from build123d import *

# Parameters (mm, degrees)
SKETCH3_W           = 6
SKETCH3_H           = 5
BOSS_EXTRUDE6_DEPTH = 6
CUT_EXTRUDE3_DEPTH  = 3


with BuildPart() as part:
    # Sketch3 → Boss-Extrude6 (new body)
    with BuildSketch(Plane.XY):
        with Locations((3, 2.5)):
            Rectangle(SKETCH3_W, SKETCH3_H)
    extrude(amount=BOSS_EXTRUDE6_DEPTH)

    # Sketch7 → Cut-Extrude3 (cut)
    with BuildSketch(Plane.ZY):
        Polygon((0, 5), (6, 3), (6, 5), align=None)
    extrude(amount=-CUT_EXTRUDE3_DEPTH, mode=Mode.SUBTRACT)


solid = part.part
Input: part model. Units: mm. Frame: model coordinates. A direction names the side the tool comes from. Round coordinates to 2 decimals unless told otherwise and drop trailing zeros. Loops run counter-clockwise (first coordinate to the right, second up) from the corner with the lowest first, then second, coordinate; pieces in that order, holes last. Notation, with made-up numbers: (-18.5, -12) -> (11.5, -12) arc R22 cw to (11.5, 18) -> close; hole circle Ø9 at (71, -39). An arc over 180 degrees is marked (long way). Answer as a JSON object with one key per item and string values. Group by question number.
1) Reachability of faces 1 (the flat face through (4, 2, 6)), 2 (the flat face through (3, 4, 4)) from +Z, -Z, +X, -X, +Y, -Y: full face, straight path, thin tool, end or side. Return the list, or none.
2) Section query B-B on z = 0.75. Output: boundary loops of the cut face in (x, y).
3) Section query C-C on x = 2.15. Output: boundary loops of the cut face in (y, z), plus the area to 3 significant figures.
4) Section query A-A on y = 3.85. Output: boundary loops of the cut face in (x, z).
5) Ray query, L1, parallel to X at y = 4.25, z = 3.75; L2, parallel to Y at x = 1.3, z = 1.75; L3, parallel to Y at x = 1, z = 1.5. Return the intervals inside material, ascending.
Reply:
{
 "1": {"face 1": "+Z, +X, -X, +Y, -Y", "face 2": "+Z, -X, +Y"},
 "2": {"outline": "(0, 0) -> (6, 0) -> (6, 5) -> (3, 5) -> (3, 4.75) -> (0, 4.75) -> close"},
 "3": {"outline": "(0, 0) -> (5, 0) -> (3, 6) -> (0, 6) -> close", "area": "24.0 mm2"},
 "4": {"outline": "(0, 0) -> (6, 0) -> (6, 6) -> (3, 6) -> (3, 3.45) -> (0, 3.45) -> close"},
 "5": {"L1": "x = 3 to 6", "L2": "y = 0 to 4.42", "L3": "y = 0 to 4.5"}
}
